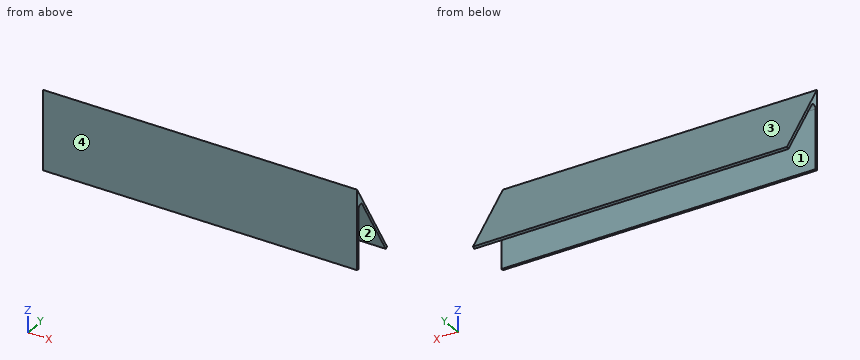
from build123d import *

# Parameters (mm, degrees)
F1_DEPTH = 100


with BuildPart() as f1:
    # F0 (on Right) → F1 (new body, symmetric)
    with BuildSketch(Plane.YZ):
        with BuildLine():
            Line((0, 50), (0, 0))
            Line((0, 0), (1.5, 0))
            Line((1.5, 0), (1.5, 37.363889))
            ThreePointArc((1.5, 37.363889), (2.966133, 39.291319), (5.214986, 38.392881))
            Line((5.214986, 38.392881), (28.713761, -0.771744))
            Line((28.713761, -0.771744), (30, 0))
            Line((30, 0), (0, 50))
        make_face()
    extrude(amount=F1_DEPTH, both=True)


solid = f1.part
For this review, take the finished solid that the model builds, in its own axes (mm). Face numbers are marked on the shaded views. Round coordinates to 2 decimals unless told otherwise and drop trailing zeros. Loops run counter-clockwise (first coordinate to the right, second up) from the corner with the lowest first, then second, coordinate; pieces in that order, holes last. Notation, with made-up numbers: (-24.5, -11) - (-11.5, -11) arc R24 ccw to (-11.5, 27) - close; hole circle Ø5 at (20.25, -25). An arc over 180 degrees is marked (long way). One line per item, written item: value. Start each with the question number.
Item 1: For L1, parallel to Y at x = -32, z = 21.5; L2, parallel to Y at x = 56.5, z = 7; L3, parallel to Z at x = -31.5, y = 3, list the stretches that pass through material, from the lowest coordinate up.
Item 2: Take a section at C-C (y = 25.5). Give the boundary of the cut face in (x, z).
Item 3: Clearance check with flat-ended pins moving along their axes: pin 1 Ø10 at (x, y) = (32, 18.5) entering from +Z; pin 2 Ø10 at (x, z) = (-22.5, 43) entering from +Y; pin 3 Ø0.8 at (x, y) = (-13.5, 0.5) entering from -Z. State where each tip first meets the part, or that it passes through.
Item 4: The part is to be moulded in two halves that separate along Y. For the marked faces 1, 2, 3 and 4, say which applies: +Y half, -Y half, draft (parallel to the pull), parting line (faces both ways), or undercut.
Item 5: Take a section at B-B (x = 74). Give the boundary of the cut face in (y, z).
Item 6: Take a section at A-A (z = 19.5). Give the boundary of the cut face in (x, y).
Answer below:
1. L1: y = 0 to 1.5, 15.35 to 17.1
1. L2: y = 0 to 1.5, 24.05 to 25.8
1. L3: z = 39.3 to 45
2. outline: (-100, 4.58) - (100, 4.58) - (100, 7.5) - (-100, 7.5) - close
3. pin 1: stops at z = 27.5
3. pin 2: stops at y = 7.2
3. pin 3: stops at z = 0
4. face 1: undercut
4. face 2: undercut
4. face 3: +Y half
4. face 4: -Y half
5. outline: (0, 0) - (1.5, 0) - (1.5, 37.36) arc R2 cw to (5.21, 38.39) - (28.71, -0.77) - (30, 0) - (0, 50) - close
6. outline: (-100, 0) - (100, 0) - (100, 1.5) - (-100, 1.5) - close; (-100, 16.55) - (100, 16.55) - (100, 18.3) - (-100, 18.3) - close
